CAD build for the part. Positions are in the model's coordinates, mm. A direction names the side the tool comes from. Give positions to 0.01 mm unless a question says otherwise; leave off trailing zeros. Loops run counter-clockwise (first coordinate to the right, second up) from the corner with the lowest first, then second, coordinate; pieces in that order, holes last.
Item 1: Saw through at C-C on x = 40.5. Give the cut face in (y, z), plus the area to 3 significant figures.
Item 2: Drop flat-ended pins along their axis: P1, Ø1, axis at x = -29.5, y = -21.5, coming from the +Z side; P2, Ø8, axis at x = -17.5, z = 20.5, coming from the +Y side; P3, Ø12, axis at x = 22.5, z = 53, coming from the +Y side. Give the stop position or say it passes through.
Item 3: Saw through at B-B on z = 15.5. Give the cut face in (x, y), plus the area to 3 significant figures.
Item 4: Saw through at D-D on x = 8. Give the number of separate pieces and of enclosed holes in the cut face, plus the area to 3 significant figures.
Item 5: Which spindle directions (+Z, -Z, +X, -X, +Y, -Y) get a long thin tool onto all of the face, cutting with end or side? Do faces 5 (the flat face through (13, -13, 101.6)), 6 (the flat face through (4.238, -24.617, 60.937)). Say none if no direction does.
Item 6: Mould opens along X. For faces 1 (the flat face through (20.771, -24.617, 70.483)), 2 (the flat face through (34, -1.587, 50.6)), 3 (the cylindrical face through (43.95, -1.35, 32.32)), 4 (the flat face through (2.674, -24.617, 42.642)) say: released by +X, released by -X, zero draft, split by the parting line, or undercut.
Item 7: Saw through at A-A on y = -21.5. Give the cut face in (x, z).
Item 8: Probe probe 1 along Z at (x, y) = (9, -19); probe 2 along X at (y, z) = (-24, 90); probe 3 along Y at (x, z) = (13, 18.5). List the from-to ranges inside material, lowest first.
from build123d import *

# Parameters (mm, degrees)
F1_DEPTH = 25.4
F3_DEPTH = 25.401
F5_W     = 22.225
F5_H     = 98.425
F6_DEPTH = 134.621
F8_DEPTH = 1.5875


with BuildPart() as f1:
    # F0 (on Front) → F1 (new body)
    with BuildSketch(Plane.XZ):
        with BuildLine():
            Line((12.7, 101.6), (12.7, 0))
            Line((12.7, 0), (76.2, 0))
            ThreePointArc((76.2, 0), (37.2138180159, 44.0069090079), (25.4, 101.6))
            Line((25.4, 101.6), (12.7, 101.6))
        make_face()
        with BuildLine():
            Line((-50.8, 0), (12.7, 0))
            Line((12.7, 0), (12.7, 101.6))
            Line((12.7, 101.6), (0, 101.6))
            ThreePointArc((0, 101.6), (-11.8138180159, 44.0069090079), (-50.8, 0))
        make_face()
    extrude(amount=F1_DEPTH)

    # F2 (on face) → F3 (cut, through all)
    with BuildSketch(Plane.XZ.offset(25.4)):
        with BuildLine():
            ThreePointArc((71.1283228984, 1.5875), (35.0396824726, 44.8338255614), (23.7282488961, 100.0125))
            Line((23.7282488961, 100.0125), (1.6717511039, 100.0125))
            ThreePointArc((1.6717511039, 100.0125), (-9.6396824726, 44.8338255614), (-45.7283228984, 1.5875))
            Line((-45.7283228984, 1.5875), (71.1283228984, 1.5875))
        make_face()
    extrude(amount=-F3_DEPTH, mode=Mode.SUBTRACT)

    # F5 (on offset) → F6 (cut, through all)
    with BuildSketch(Plane.YZ.offset(83.82)):
        with Locations((-12.7, 50.8)):
            Rectangle(F5_W, F5_H)
    extrude(amount=-F6_DEPTH, mode=Mode.SUBTRACT)

    # F7 (on face) → F8 (join)
    with BuildSketch(Plane.XZ.offset(25.4)):
        with BuildLine():
            Line((13.9308617211, 91.7459002665), (23.7282488961, 100.0125))
            Line((23.7282488961, 100.0125), (21.2665254539, 100.0125))
            Line((21.2665254539, 100.0125), (12.7, 92.784446666))
            Line((12.7, 92.784446666), (12.7, 90.7073538669))
            Line((12.7, 90.7073538669), (23.203703887, 81.8447954927))
            Line((23.203703887, 81.8447954927), (12.7, 75.4199183699))
            Line((12.7, 75.4199183699), (12.7, 73.5589856846))
            Line((12.7, 73.5589856846), (14.2211719622, 74.4894520272))
            Line((14.2211719622, 74.4894520272), (24.4823150631, 80.7659602259))
            ThreePointArc((24.4823150631, 80.7659602259), (24.3465871841, 81.9135246636), (24.2223606039, 83.0623910408))
            Line((24.2223606039, 83.0623910408), (13.9308617211, 91.7459002665))
        make_face()
        with BuildLine():
            Line((12.7, 90.7073538669), (12.7, 92.784446666))
            Line((12.7, 92.784446666), (4.1334745461, 100.0125))
            Line((4.1334745461, 100.0125), (1.6717511039, 100.0125))
            Line((1.6717511039, 100.0125), (11.4691382789, 91.7459002665))
            Line((11.4691382789, 91.7459002665), (1.1776393961, 83.0623910408))
            ThreePointArc((1.1776393961, 83.0623910408), (1.0534128159, 81.9135246636), (0.9176849369, 80.7659602259))
            Line((0.9176849369, 80.7659602259), (11.1788280378, 74.4894520272))
            Line((11.1788280378, 74.4894520272), (-1.7401008163, 66.5872366432))
            ThreePointArc((-1.7401008163, 66.5872366432), (-1.8224554679, 66.2637756063), (-1.9057456257, 65.9405541952))
            Line((-1.9057456257, 65.9405541952), (-0.7461259732, 65.3342957957))
            Line((-0.7461259732, 65.3342957957), (12.7, 73.5589856846))
            Line((12.7, 73.5589856846), (12.7, 75.4199183699))
            Line((12.7, 75.4199183699), (2.196296113, 81.8447954927))
            Line((2.196296113, 81.8447954927), (12.7, 90.7073538669))
        make_face()
        with BuildLine():
            Line((27.1401008163, 66.5872366432), (14.2211719622, 74.4894520272))
            Line((14.2211719622, 74.4894520272), (12.7, 73.5589856846))
            Line((12.7, 73.5589856846), (26.1461259732, 65.3342957957))
            Line((26.1461259732, 65.3342957957), (27.3057456257, 65.9405541952))
            ThreePointArc((27.3057456257, 65.9405541952), (27.2224554679, 66.2637756063), (27.1401008163, 66.5872366432))
        make_face()
        with BuildLine():
            Line((12.7, 56.5131896629), (12.7, 58.3045539367))
            Line((12.7, 58.3045539367), (-0.7461259732, 65.3342957957))
            Line((-0.7461259732, 65.3342957957), (-2.3251365904, 64.3684508614))
            Line((-2.3251365904, 64.3684508614), (10.9867856194, 57.4088717998))
            Line((10.9867856194, 57.4088717998), (-8.5307429304, 47.204952269))
            ThreePointArc((-8.5307429304, 47.204952269), (-8.7388685778, 46.7490885521), (-8.9489724475, 46.2941331944))
            Line((-8.9489724475, 46.2941331944), (-7.6357223304, 45.8815119005))
            Line((-7.6357223304, 45.8815119005), (12.7, 56.5131896629))
        make_face()
        with BuildLine():
            Line((26.1461259732, 65.3342957957), (12.7, 58.3045539367))
            Line((12.7, 58.3045539367), (12.7, 56.5131896629))
            Line((12.7, 56.5131896629), (33.0357223304, 45.8815119005))
            Line((33.0357223304, 45.8815119005), (34.3489724475, 46.2941331944))
            ThreePointArc((34.3489724475, 46.2941331944), (34.1388685778, 46.7490885521), (33.9307429304, 47.204952269))
            Line((33.9307429304, 47.204952269), (14.4132143806, 57.4088717998))
            Line((14.4132143806, 57.4088717998), (27.7251365904, 64.3684508614))
            Line((27.7251365904, 64.3684508614), (26.1461259732, 65.3342957957))
        make_face()
        with BuildLine():
            Line((12.7, 37.8147295273), (12.7, 39.4920572546))
            Line((12.7, 39.4920572546), (-7.6357223304, 45.8815119005))
            Line((-7.6357223304, 45.8815119005), (-9.6396824726, 44.8338255614))
            Line((-9.6396824726, 44.8338255614), (10.030783861, 38.653393391))
            Line((10.030783861, 38.653393391), (-18.3805162111, 29.7266038582))
            ThreePointArc((-18.3805162111, 29.7266038582), (-18.6444962244, 29.3426124449), (-18.9100250772, 28.9596904146))
            Line((-18.9100250772, 28.9596904146), (-17.1145505748, 28.4470407091))
            Line((-17.1145505748, 28.4470407091), (12.7, 37.8147295273))
        make_face()
        with BuildLine():
            Line((33.0357223304, 45.8815119005), (12.7, 39.4920572546))
            Line((12.7, 39.4920572546), (12.7, 37.8147295273))
            Line((12.7, 37.8147295273), (42.5145505748, 28.4470407091))
            Line((42.5145505748, 28.4470407091), (44.3100250772, 28.9596904146))
            ThreePointArc((44.3100250772, 28.9596904146), (44.0444962244, 29.3426124449), (43.7805162111, 29.7266038582))
            Line((43.7805162111, 29.7266038582), (15.369216139, 38.653393391))
            Line((15.369216139, 38.653393391), (35.0396824726, 44.8338255614))
            Line((35.0396824726, 44.8338255614), (33.0357223304, 45.8815119005))
        make_face()
        with BuildLine():
            Line((42.5145505748, 28.4470407091), (12.7, 19.9342934931))
            Line((12.7, 19.9342934931), (12.7, 18.2701443298))
            Line((12.7, 18.2701443298), (71.1283228984, 1.5875))
            ThreePointArc((71.1283228984, 1.5875), (69.3505916333, 2.9065647427), (67.5984969335, 4.2594965256))
            Line((67.5984969335, 4.2594965256), (15.6142096044, 19.1022189114))
            Line((15.6142096044, 19.1022189114), (45.2894191126, 27.575181014))
            Line((45.2894191126, 27.575181014), (42.5145505748, 28.4470407091))
        make_face()
        with BuildLine():
            Line((12.7, 18.2701443298), (12.7, 19.9342934931))
            Line((12.7, 19.9342934931), (-17.1145505748, 28.4470407091))
            Line((-17.1145505748, 28.4470407091), (-19.8894191126, 27.575181014))
            Line((-19.8894191126, 27.575181014), (9.7857903956, 19.1022189114))
            Line((9.7857903956, 19.1022189114), (-42.1984969335, 4.2594965256))
            ThreePointArc((-42.1984969335, 4.2594965256), (-43.9505916333, 2.9065647427), (-45.7283228984, 1.5875))
            Line((-45.7283228984, 1.5875), (12.7, 18.2701443298))
        make_face()
        with BuildLine():
            Line((-19.8894191126, 27.575181014), (-17.1145505748, 28.4470407091))
            Line((-17.1145505748, 28.4470407091), (-18.9100250772, 28.9596904146))
            ThreePointArc((-18.9100250772, 28.9596904146), (-19.3971779809, 28.2656360226), (-19.8894191126, 27.575181014))
        make_face()
        with BuildLine():
            Line((34.3489724475, 46.2941331944), (33.0357223304, 45.8815119005))
            Line((33.0357223304, 45.8815119005), (35.0396824726, 44.8338255614))
            ThreePointArc((35.0396824726, 44.8338255614), (34.6917714104, 45.5627703936), (34.3489724475, 46.2941331944))
        make_face()
        with BuildLine():
            Line((44.3100250772, 28.9596904146), (42.5145505748, 28.4470407091))
            Line((42.5145505748, 28.4470407091), (45.2894191126, 27.575181014))
            ThreePointArc((45.2894191126, 27.575181014), (44.7971779809, 28.2656360226), (44.3100250772, 28.9596904146))
        make_face()
        with BuildLine():
            Line((-9.6396824726, 44.8338255614), (-7.6357223304, 45.8815119005))
            Line((-7.6357223304, 45.8815119005), (-8.9489724475, 46.2941331944))
            ThreePointArc((-8.9489724475, 46.2941331944), (-9.2917714104, 45.5627703936), (-9.6396824726, 44.8338255614))
        make_face()
        with BuildLine():
            ThreePointArc((27.7251365904, 64.3684508614), (27.5126695085, 65.153763147), (27.3057456257, 65.9405541952))
            Line((27.3057456257, 65.9405541952), (26.1461259732, 65.3342957957))
            Line((26.1461259732, 65.3342957957), (27.7251365904, 64.3684508614))
        make_face()
        with BuildLine():
            Line((-2.3251365904, 64.3684508614), (-0.7461259732, 65.3342957957))
            Line((-0.7461259732, 65.3342957957), (-1.9057456257, 65.9405541952))
            ThreePointArc((-1.9057456257, 65.9405541952), (-2.1126695085, 65.153763147), (-2.3251365904, 64.3684508614))
        make_face()
    extrude(amount=-F8_DEPTH)


solid = f1.part
Results below:
1. outline: (-25.4, 0) - (0, 0) - (0, 1.59) - (-25.4, 1.59) - close; (-25.4, 10.33) - (-23.81, 10.33) - (-23.81, 12) - (-25.4, 12) - close; (-25.4, 26.21) - (-23.81, 26.21) - (-23.81, 27.87) - (-25.4, 27.87) - close; (-25.4, 29.08) - (-23.81, 29.08) - (-23.81, 30.76) - (-25.4, 30.76) - close; (-25.4, 34.8) - (-23.81, 34.8) - (-23.81, 37.91) - (-25.4, 37.91) - close; (-1.59, 34.8) - (0, 34.8) - (0, 37.91) - (-1.59, 37.91) - close
1. area: 58.1 mm2
2. P1: stops at z = 1.59
2. P2: passes through
2. P3: stops at y = -23.81
3. outline: (-32.08, -25.4) - (-29.88, -25.4) - (-29.88, -23.81) - (-32.08, -23.81) - close; (-32.08, -1.59) - (-29.88, -1.59) - (-29.88, 0) - (-32.08, 0) - close; (-2.83, -25.4) - (3, -25.4) - (3, -23.81) - (-2.83, -23.81) - close; (22.4, -25.4) - (28.23, -25.4) - (28.23, -23.81) - (22.4, -23.81) - close; (55.28, -25.4) - (57.48, -25.4) - (57.48, -23.81) - (55.28, -23.81) - close; (55.28, -1.59) - (57.48, -1.59) - (57.48, 0) - (55.28, 0) - close
3. area: 32.5 mm2
4. separate pieces: 12
4. enclosed holes: 0
4. area: 109 mm2
5. face 5: +Z, +X, -X, +Y, -Y
5. face 6: +Y, -Y
6. face 1: undercut
6. face 2: zero draft
6. face 3: released by +X
6. face 4: undercut
7. outline: (-50.8, 0) - (76.2, 0) arc R113.78 cw to (73.86, 1.59) - (-48.46, 1.59) arc R113.78 cw to start; (0, 101.6) arc R113.78 cw to (0.08, 100.01) - (25.32, 100.01) arc R113.78 cw to (25.4, 101.6) - close
8. probe 1: z = 0 to 1.59, 100.01 to 101.6
8. probe 2: x = 0.09 to 1.68, 9.4 to 11.86, 13.54 to 16, 23.72 to 25.31
8. probe 3: y = -25.4 to -23.81
